Part model, mm, in its own coordinate system. Coordinates: 2 decimals unless noted, no trailing zeros. Order: outer loops, then holes, each group sorted by start corner. A loop starts at its lowest first (then second) coordinate and runs counter-clockwise, first axis right, second up.
Autodesk Inventor part; units mm, degrees
ref_plane "工作平面1" through (10, 18, 0) normal (-0.3855, -0.6524, -0.6524) x (0.8609, 0, -0.5087)
ref_plane "YZ Plane" through (0, 0, 0) normal (1, 0, 0) x (0, 1, 0)
ref_plane "XZ Plane" through (0, 0, 0) normal (0, 1, 0) x (-1, 0, 0)
sketch "草圖1" plane through (0, 0, 0) normal (0, 1, 0) x (-1, 0, 0)
  line L0 (0, 0) -> (-54, 0)
  line L1 (-54, 0) -> (-54, -36)
  line L2 (-54, -36) -> (0, -36)
  line L3 (0, -36) -> (0, 0)
  dimension "d0" = 54
  dimension "d1" = 36
extrude "擠出1" add sketch "草圖1" along normal mid plane 36
sketch "草圖2" plane through (0, 18, 0) normal (0, 1, 0) x (1, 0, 0)
  line L0 (0, 0) -> (54, 0)
  line L1 (10, 0) -> (54, 6)
  line L2 (54, 0) -> (54, 36)
  dimension "d4" = 10
  dimension "d5" = 30
extrude "擠出2" cut sketch "草圖2" against normal blind 40
sketch "草圖3" plane through (54, -18, -36) normal (1, 0, 0) x (0, 0, -1)
  line L0 (-30, 16) -> (-10, 36)
  line L1 (0, 36) -> (-36, 36)
  line L2 (-30, 36) -> (-30, 0)
  point P0 (-36, 18)
  dimension "d8" = 20
  dimension "d9" = 20
ref_plane "工作平面1" through (10, 18, 0) normal (-0.3855, -0.6524, -0.6524) x (0.8609, 0, -0.5087)
sketch "草圖4" plane through (10, 18, 0) normal (-0.3855, -0.6524, -0.6524) x (0.8609, 0, -0.5087)
  line L0 (-15.1543, -12.3218) -> (93.717, -12.3218)
  line L1 (93.717, -12.3218) -> (93.717, 28.8166)
  line L2 (93.717, 28.8166) -> (-15.1543, 28.8166)
  line L3 (-15.1543, 28.8166) -> (-15.1543, -12.3218)
  point P0 (-8.6093, 10.3219)
extrude "擠出3" cut sketch "草圖4" against normal blind 40
mirror "鏡射1" about plane through (0, 0, 0) normal (0, 1, 0) of "擠出3"
properties part number "1"
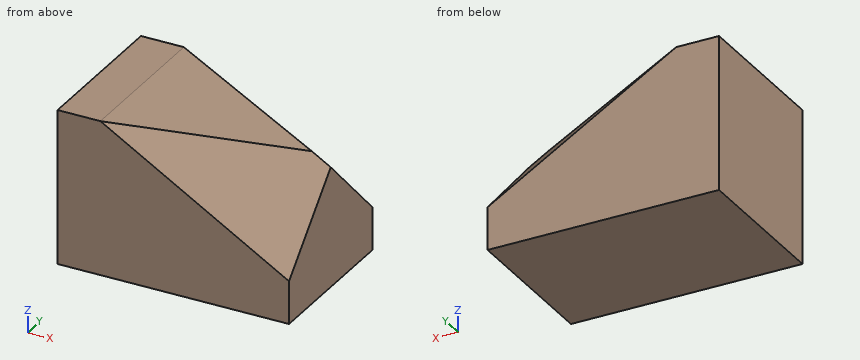
Q1. Cut at B-B on x = 38.5. Write the cut outline in (y, z).
Results list:
outline: (-18, -36) - (18, -36) - (18, -16.84) - (5.04, -3.89) - (-5.04, -3.89) - (-18, -16.84) - close
Q2. Wall check: line 1 along Z through (x, y) = (45, 15); line 2 along Z through (x, y) = (14.5, 6.5); line 3 along X through (y, z) = (-14, -13.5). Give the ranges that are in metal, low to high.
Results list:
line 1: z = -36 to -17.68
line 2: z = -36 to -0.61
line 3: x = 0 to 39.61
Q3. Cut at A-A on y = 13.5. Write the cut outline in (x, z), and give its area (3 significant figures).
Results list:
outline: (0, -36) - (54, -36) - (54, -21.5) - (19.89, -1.35) - (10, 0) - (0, 0) - close
area: 1,550 mm2
